Design review of the part shown in the three views and the two pictorial views. Dimensions are in mm from the part's minimum x, y and z. Give positions to 0.01 mm unless a question says otherwise; leave off trailing zeros. Loops run counter-clockwise (first coordinate to the right, second up) from the corner with the lowest first, then second, coordinate; pieces in that order, holes last.
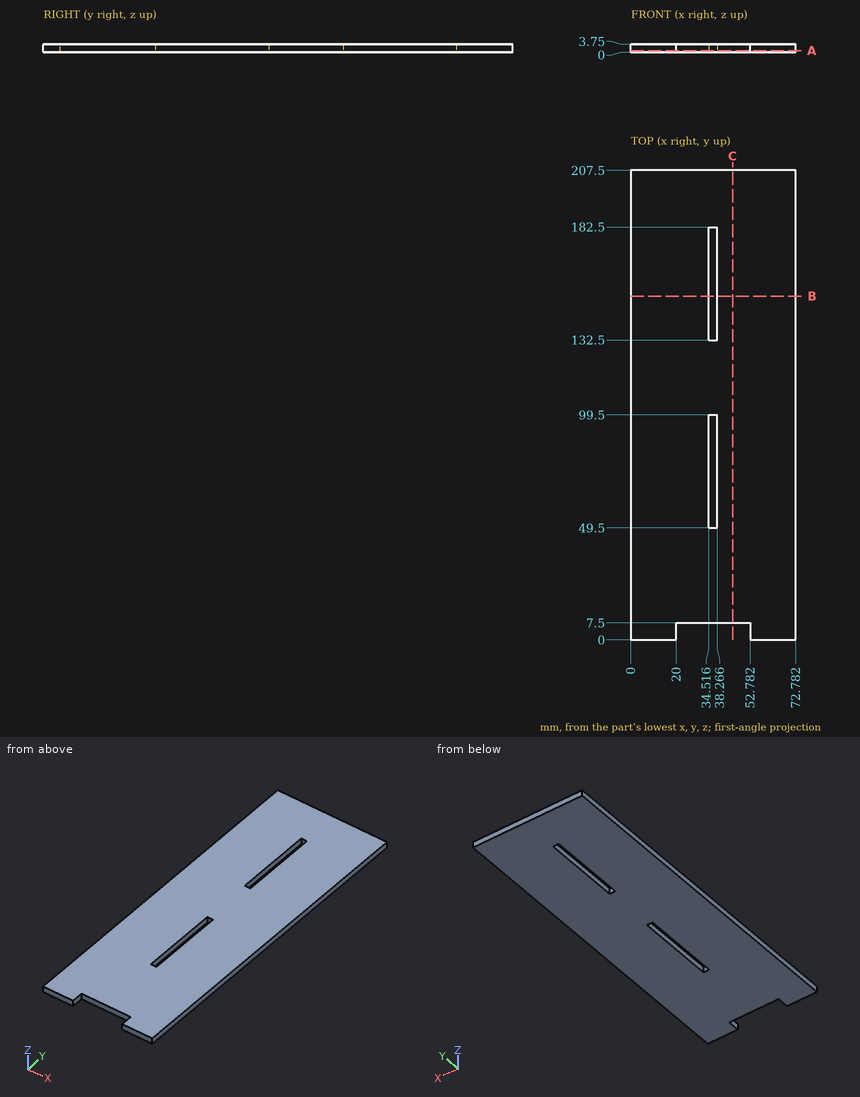
Q1. Wall thickness on line 1 (X direction, y = 77, z = 1.5); line 2 (Y direction, x = 20.5, z = 1.7): over which ranges is each line inside the solid? List them lowest first.
Results:
line 1: x = 0 to 34.52, 38.27 to 72.78
line 2: y = 7.5 to 207.5
Q2. Take a section at A-A (z = 0.8). Give the boundary of the cut face in (x, y).
Results:
outline: (0, 0) - (20, 0) - (20, 7.5) - (52.78, 7.5) - (52.78, 0) - (72.78, 0) - (72.78, 207.5) - (0, 207.5) - close; hole (34.52, 49.5) - (38.27, 49.5) - (38.27, 99.5) - (34.52, 99.5) - close; hole (34.52, 132.5) - (38.27, 132.5) - (38.27, 182.5) - (34.52, 182.5) - close
Q3. Take a section at B-B (y = 152). Give the boundary of the cut face in (x, z).
Results:
outline: (0, 0) - (34.52, 0) - (34.52, 3.75) - (0, 3.75) - close; (38.27, 0) - (72.78, 0) - (72.78, 3.75) - (38.27, 3.75) - close
Q4. Take a section at C-C (x = 45). Give the boundary of the cut face in (y, z), plus the area to 3 significant figures.
Results:
outline: (7.5, 0) - (207.5, 0) - (207.5, 3.75) - (7.5, 3.75) - close
area: 750 mm2
Q5. Insertion check: pin 1 (6 mm diameter, centred on x = 41, y = 156.5, fed in from -Z); pin 2 (1.1 mm diameter, centred on x = 36.5, z = 1.5, fed in from -Y). Each pin has a flat end and moves straight along its axis. Give the tip position at first contact, or say it passes through.
Results:
pin 1: stops at z = 0
pin 2: stops at y = 7.5
